Verification items for the finished model (mm, model axes). A direction names the side the tool comes from. Give positions to 0.01 mm unless a question says otherwise; leave off trailing zeros. Loops run counter-clockwise (first coordinate to the right, second up) from the corner with the lowest first, then second, coordinate; pieces in that order, holes last. Notation, with made-up numbers: (36.5, 32.25) -> (74.5, 32.25) arc R27 ccw to (74.5, 62.25) -> close; hole circle Ø4 at (-4.5, -11). An arc over 180 degrees is marked (long way). Answer in a Markdown table with one row per item. Add a question column.
Q1. Section check C-C on y = -77.5. Enter the section's corners in (x, z), and give its area (3 significant figures).
Q2. Set-up check for faces 1 (the face through (-5.506, -250.444, 24.796)), 2 (the face through (3, 50.8, 3)): record each of +Z, -Z, +X, -X, +Y, -Y from which the full face is reachable in a straight line by a thin tool's end or side.
Q3. Section check A-A on z = 0. Enter the section's corners in (x, y).
Q4. Release check for a two-part mould opening along Y. For faces 3 (the face through (101.632, -509.364, 32.005)), 4 (the face through (-27.53, -531.58, 123.98)), 5 (the face through (-2, -533.4, 2)) record: pulls with the +Y half, pulls with the -Y half, needs draft (parallel to the pull), parting line crosses it, or undercut.
Q5. Section check B-B on x = 0. Enter the section's corners in (y, z), and give its area (3 significant figures).
Q6. Gauge pin test, flat end, axial feed: P1, Ø1, axis at x = -166.5, z = 75, coming from the -Y side. Record the tip position at first contact, or that the pin passes through.
Q7. Material ranges on probe 1 along Y at (x, z) = (31, 14); probe 2 along Y at (x, z) = (5, -188); probe 3 along Y at (x, z) = (-114.5, -2), recorded low to high.
Autodesk Inventor part; units mm, degrees
ref_plane "YZ Plane" through (0, 0, 0) normal (1, 0, 0) x (0, 1, 0)
ref_plane "XZ Plane" through (0, 0, 0) normal (0, 1, 0) x (-1, 0, 0)
ref_plane "XY Plane" through (0, 0, 0) normal (0, 0, 1) x (1, 0, 0)
sketch "Sketch1" plane through (0, 0, 0) normal (0, 1, 0) x (-1, 0, 0)
  circle A0 centre (0, 0) radius 228.6
  dimension "d0" = 457.2
extrude "Extrusion1" add sketch "Sketch1" along normal blind 50.8
fillet "Fillet1" radius 15.85 1 edges at (228.6, 50.8, 0)
sketch "Sketch2" plane through (0, 0, 0) normal (0, -1, 0) x (1, 0, 0)
  circle A0 centre (0, 0) radius 25.4
  dimension "d4" = 50.8
extrude "Extrusion2" add sketch "Sketch2" along normal blind 508
sketch "Sketch3" plane through (0, -508, 0) normal (0, -1, 0) x (1, 0, 0)
  circle A0 centre (0, 0) radius 127
  dimension "d7" = 254
extrude "Extrusion3" add sketch "Sketch3" along normal blind 25.4
chamfer "Chamfer1" distance 21.8125 angle 45 1 edges at (-127, -508, 0)
properties part number "Stool" material "Aluminum 6061, Welded"
Taken from the geometry:
| question | item | result |
|---|---|---|
| 1 | outline | circle Ø50.8 at (0, 0) |
| 1 | area | 2,030 mm² |
| 2 | face 1 | none |
| 2 | face 2 | +Z, -Z, +X, -X, +Y |
| 3 | outline | (-228.6, 0) -> (-25.4, 0) -> (-25.4, -508) -> (-105.19, -508) -> (-127, -529.81) -> (-127, -533.4) -> (127, -533.4) -> (127, -529.81) -> (105.19, -508) -> (25.4, -508) -> (25.4, 0) -> (228.6, 0) -> (228.6, 34.95) arc R15.85 ccw to (212.75, 50.8) -> (-212.75, 50.8) arc R15.85 ccw to (-228.6, 34.95) -> close |
| 4 | face 3 | undercut |
| 4 | face 4 | needs draft |
| 4 | face 5 | pulls with the -Y half |
| 5 | outline | (-533.4, -127) -> (-529.81, -127) -> (-508, -105.19) -> (-508, -25.4) -> (0, -25.4) -> (0, -228.6) -> (34.95, -228.6) arc R15.85 ccw to (50.8, -212.75) -> (50.8, 212.75) arc R15.85 ccw to (34.95, 228.6) -> (0, 228.6) -> (0, 25.4) -> (-508, 25.4) -> (-508, 105.19) -> (-529.81, 127) -> (-533.4, 127) -> close |
| 5 | area | 54,900 mm² |
| 6 | P1 | stops at y = 0 |
| 7 | probe 1 | y = -533.4 to -508, 0 to 50.8 |
| 7 | probe 2 | y = 0 to 50.8 |
| 7 | probe 3 | y = -533.4 to -517.33, 0 to 50.8 |
